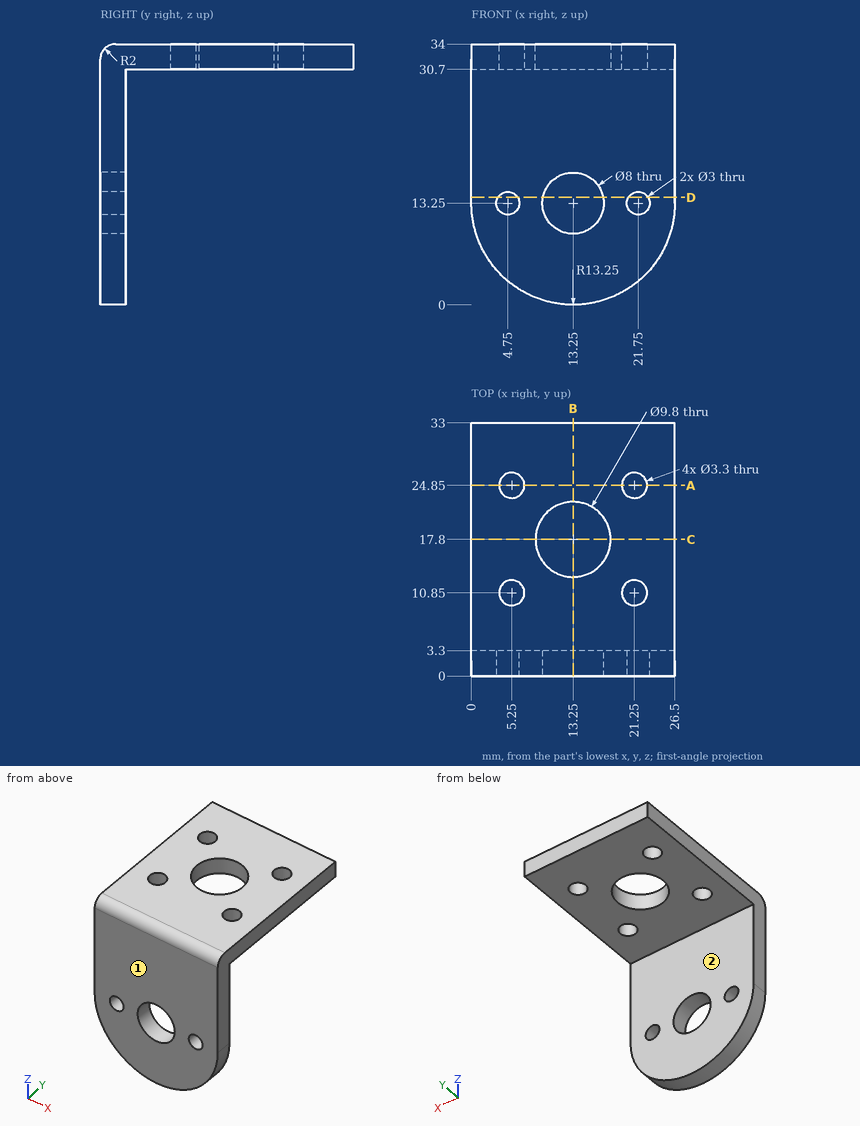
Could you check a few things on this drawing? It's one solid part, dimensions in mm from its lowest x, y, z. A direction names the side the tool comes from. Round coordinates to 2 decimals unless told otherwise and drop trailing zeros. Write each loop counter-clockwise with the first axis right and the second up, starting at its lowest first coordinate (ties: lowest second). Pieces come first, ordered by that corner, then holes.
Q1. If we section it at A-A on y = 24.85: Write out the boundary of the cut face in (x, z), plus the area to 3 significant figures.
Q2. If we section it at B-B on x = 13.25: Write out the boundary of the cut face in (y, z), plus the area to 3 significant figures.
Q3. If we section it at C-C on y = 17.8: Write out the boundary of the cut face in (x, z).
Q4. Will these pins go through, and if not, where does the flat tip stop? P1, Ø8, axis at y = 4.5, z = 16.5, coming from the +X side; P2, Ø8, axis at x = 15.5, z = 15.5, coming from the +Y side; P3, Ø2.5, axis at x = 5.25, y = 10.85, coming from the -Z side; P4, Ø8, axis at y = 5, z = 7.5, coming from the +X side.
Q5. If we section it at D-D on z = 14: Write out the boundary of the cut face in (x, y), plus the area to 3 significant figures.
Q6. Which directions (+Z, -Z, +X, -X, +Y, -Y) give clear straight access to the entire face, cutting with the end or side of a thin tool? Please do the marked faces 1 and 2.
Q7. Please list where these lines run through material, in increasing order: probe 1 along Y at (x, z) = (5.25, 31.65); probe 2 along X at (y, z) = (1.1, 13.25); probe 3 along Y at (x, z) = (21.25, 33.3).
Answer below:
1. outline: (0, 30.7) - (3.6, 30.7) - (3.6, 34) - (0, 34) - close; (6.9, 30.7) - (19.6, 30.7) - (19.6, 34) - (6.9, 34) - close; (22.9, 30.7) - (26.5, 30.7) - (26.5, 34) - (22.9, 34) - close
1. area: 65.7 mm2
2. outline: (0, 0) - (3.3, 0) - (3.3, 9.25) - (0, 9.25) - close; (0, 17.25) - (3.3, 17.25) - (3.3, 30.7) - (12.9, 30.7) - (12.9, 34) - (2, 34) arc R2 ccw to (0, 32) - close; (22.7, 30.7) - (33, 30.7) - (33, 34) - (22.7, 34) - close
2. area: 151 mm2
3. outline: (0, 30.7) - (8.35, 30.7) - (8.35, 34) - (0, 34) - close; (18.15, 30.7) - (26.5, 30.7) - (26.5, 34) - (18.15, 34) - close
4. P1: stops at x = 26.5
4. P2: stops at y = 3.3
4. P3: passes through
4. P4: stops at x = 26.33
5. outline: (0, 0) - (3.45, 0) - (3.45, 3.3) - (0, 3.3) - close; (6.05, 0) - (9.32, 0) - (9.32, 3.3) - (6.05, 3.3) - close; (17.18, 0) - (20.45, 0) - (20.45, 3.3) - (17.18, 3.3) - close; (23.05, 0) - (26.5, 0) - (26.5, 3.3) - (23.05, 3.3) - close
5. area: 44.4 mm2
6. face 1: +Z, -Z, +X, -X, -Y
6. face 2: -Z, +X, -X, +Y
7. probe 1: y = 0 to 9.2, 12.5 to 23.2, 26.5 to 33
7. probe 2: x = 0 to 3.25, 6.25 to 9.25, 17.25 to 20.25, 23.25 to 26.5
7. probe 3: y = 0.48 to 9.2, 12.5 to 23.2, 26.5 to 33
